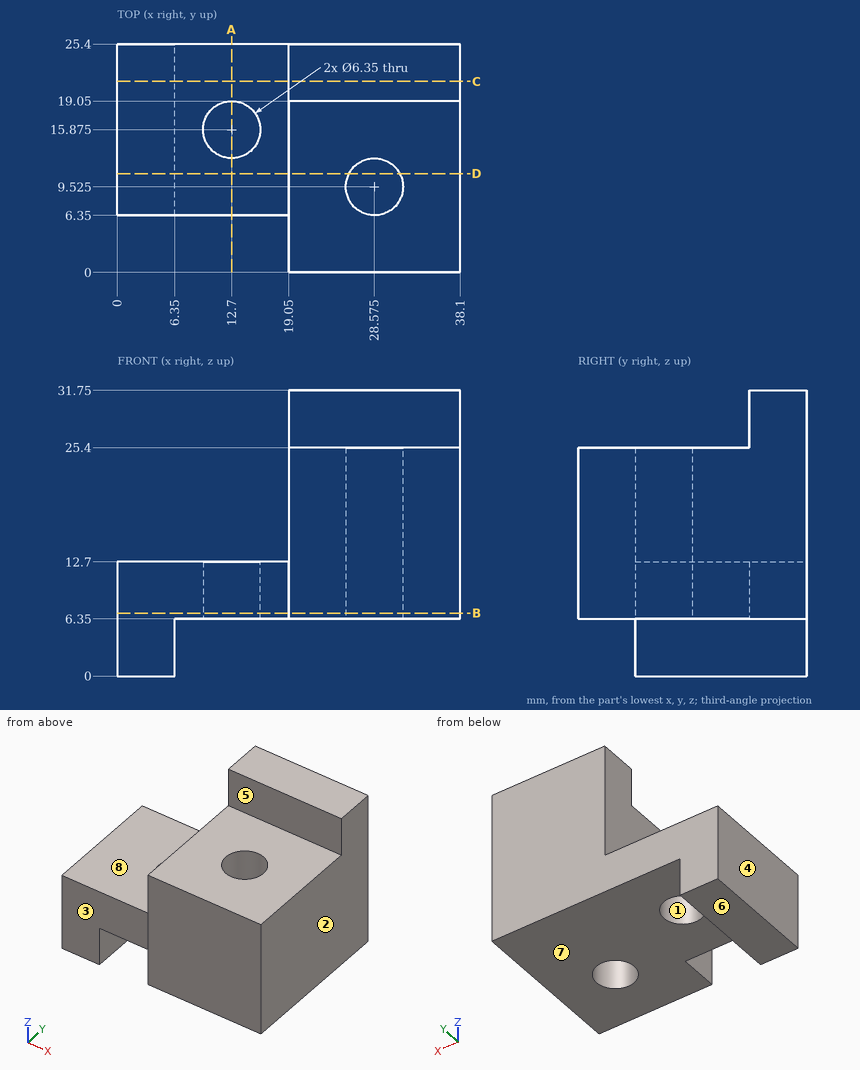
Geometry: see drawing. Coordinates: mm, zero at the bounding-box minimum. A direction names the side the tool comes from. Give positions to 0.01 mm unless a question says otherwise; leave off trailing zeros. Loops run counter-clockwise (first coordinate to the right, second up) from the corner with the lowest first, then second, coordinate; pieces in that order, holes last. Notation, with made-up numbers: (-17.75, 81.25) - (19.25, 81.25) arc R25 cw to (19.25, 118.25) - close; hole circle Ø1 at (32, 63.25). An arc over 180 degrees is marked (long way). Use CSV: the item, a comma, the result in double quotes. Start each with the question number.
Item 1: Mould query, pull axis Y, two halves, no side actions, for the marked faces 1, 2 and 3. Classes: pulls with the +Y half, pulls with the -Y half, needs draft (parallel to the pull), parting line crosses it, or undercut.
Item 2: Line query: line 1 (Y direction, x = 12.7, z = 8); line 2 (X direction, y = 14.5, z = 16); line 3 (Z direction, x = 28, y = 2). Output: solid intervals per line, ascending.
Item 3: Contact query for flat-ended pins moving along their axis: P1, Ø2, axis at x = 23, y = 9, coming from the -Z side; P2, Ø9.5, axis at x = 29, y = 12, coming from the +Z side; P3, Ø3, axis at y = 12, z = 22, coming from the -X side. Output: stop coordinate, or through.
Item 4: Section A-A on x = 12.7. Return loops of the section in (y, z).
Item 5: Section D-D on y = 11. Return loops of the section in (x, z), then the cut area to 3 significant figures.
Item 6: Section B-B on z = 7. Return loops of the section in (x, y) (3 decimals).
Item 7: Reachability of the marked faces 4, 5, 6, 7 and 8 from +Z, -Z, +X, -X, +Y, -Y: full face, straight path, thin tool, end or side. Return the list, or none.
Item 8: Section C-C on y = 21.25. Return loops of the section in (x, z), then the cut area to 3 significant figures.
Ans:
1,face 1,"undercut"
1,face 2,"needs draft"
1,face 3,"pulls with the -Y half"
2,line 1,"y = 6.35 to 12.7, 19.05 to 25.4"
2,line 2,"x = 19.05 to 38.1"
2,line 3,"z = 6.35 to 25.4"
3,P1,"stops at z = 6.35"
3,P2,"stops at z = 25.4"
3,P3,"stops at x = 19.05"
4,outline,"(6.35, 6.35) - (12.7, 6.35) - (12.7, 12.7) - (6.35, 12.7) - close; (19.05, 6.35) - (25.4, 6.35) - (25.4, 12.7) - (19.05, 12.7) - close"
5,outline,"(0, 0) - (6.35, 0) - (6.35, 6.35) - (25.76, 6.35) - (25.76, 25.4) - (19.05, 25.4) - (19.05, 12.7) - (0, 12.7) - close; (31.39, 6.35) - (38.1, 6.35) - (38.1, 25.4) - (31.39, 25.4) - close"
5,area,"417 mm2"
6,outline,"(0, 6.35) - (19.05, 6.35) - (19.05, 0) - (38.1, 0) - (38.1, 25.4) - (0, 25.4) - close; hole circle Ø6.35 at (12.7, 15.875); hole circle Ø6.35 at (28.575, 9.525)"
7,face 4,"+Z, -Z, -X, +Y, -Y"
7,face 5,"+Z, +X, -X, -Y"
7,face 6,"-Z, +X, -X, +Y, -Y"
7,face 7,"-Z, +X, +Y, -Y"
7,face 8,"+Z, -X, +Y, -Y"
8,outline,"(0, 0) - (6.35, 0) - (6.35, 6.35) - (38.1, 6.35) - (38.1, 31.75) - (19.05, 31.75) - (19.05, 12.7) - (0, 12.7) - close"
8,area,"645 mm2"
